Geometry check sheet. Reference: the model listing, model coordinates, mm. Give positions to 0.01 mm unless a question says otherwise; leave off trailing zeros. Write each loop counter-clockwise with the first axis right and the second up, starting at its lowest first coordinate (ties: lowest second). Pieces come first, ordered by that corner, then holes. Notation, with made-up numbers: M -29.75,89 L 27.25,89 A27 cw 27.25,119 Z; hole C 3,45 d5. An arc over 180 degrees is marked long. One line per item, written item: value. Start each with the question number.
1. Cross-section at C-C on z = -24. Record the cut outline in (x, y), then the cut area to 3 significant figures.
2. Scan line: line 1 (X direction, y = 11.5, z = -6). Record every from-to range of solid material in increasing order.
3. Cross-section at B-B on x = 29. Record the cut outline in (y, z).
4. Release check for a two-part mould opening along Z. For faces 1 (the face through (3.753, 11.154, -25.627)), 2 (the face through (17, 11, 0)), 3 (the face through (17, 22, -15)) record: pulls with the +Z half, pulls with the -Z half, needs draft (parallel to the pull), parting line crosses it, or undercut.
5. Gauge pin test, flat end, axial feed: pin 1 (3.5 mm diameter, centred on x = 29, z = -6, fed in from -Y). Record the tip position at first contact, or that the pin passes through.
6. Cross-section at A-A on y = 16.75. Record the cut outline in (x, z).
from build123d import *

# Parameters (mm, degrees)
SKETCH2_W           = 34
SKETCH2_H           = 22
BOSS_EXTRUDE1_DEPTH = 30
SKETCH3_R           = 2.05
CUT_EXTRUDE1_DEPTH  = 30


with BuildPart() as part:
    # Sketch2 → Boss-Extrude1 (new body)
    with BuildSketch(Plane.XY):
        with Locations((17, 11)):
            Rectangle(SKETCH2_W, SKETCH2_H)
    extrude(amount=-BOSS_EXTRUDE1_DEPTH)

    # Sketch3 → Cut-Extrude1 (cut)
    with BuildSketch(Plane(origin=(0, 22, 0), x_dir=(1, 0, 0), z_dir=(0, 1, 0))):
        with Locations(Location((29, 6, 0), (0, 0, 270))):
            Circle(SKETCH3_R)
        with Locations(Location((5, 6, 0), (0, 0, 270))):
            Circle(SKETCH3_R)
        with Locations(Location((5, 24, 0), (0, 0, 270))):
            Circle(SKETCH3_R)
        with Locations(Location((29, 24, 0), (0, 0, 270))):
            Circle(SKETCH3_R)
    extrude(amount=-CUT_EXTRUDE1_DEPTH, mode=Mode.SUBTRACT)


solid = part.part
Report:
1. outline: M 0,0 L 2.95,0 L 2.95,22 L 0,22 Z; M 7.05,0 L 26.95,0 L 26.95,22 L 7.05,22 Z; M 31.05,0 L 34,0 L 34,22 L 31.05,22 Z
1. area: 568 mm^2
2. line 1: x = 0 to 2.95, 7.05 to 26.95, 31.05 to 34
3. outline: M 0,-30 L 22,-30 L 22,-26.05 L 0,-26.05 Z; M 0,-21.95 L 22,-21.95 L 22,-8.05 L 0,-8.05 Z; M 0,-3.95 L 22,-3.95 L 22,0 L 0,0 Z
4. face 1: undercut
4. face 2: pulls with the +Z half
4. face 3: needs draft
5. pin 1: passes through
6. outline: M 0,-30 L 34,-30 L 34,0 L 0,0 Z; hole C 5,-24 d4.1; hole C 5,-6 d4.1; hole C 29,-24 d4.1; hole C 29,-6 d4.1
